```python
from build123d import *

# Parameters (mm, degrees)
F0_R        = 3.15
F1_DEPTH    = 6.5
F2_T1_DEPTH = 23.3593154951
F2_T3_DEPTH = 23.1607876028
F4_R        = 2


# Not quite as in the source:
# - a fillet or chamfer that OpenCascade refuses, or shapes differently, is made with other operations: its cross-section is extruded or revolved along the edge and cut away or added
# - two fillets or chamfers of one size are made in one step


with BuildPart() as f1:
    # F0 (on Top) → F1 (new body, symmetric)
    with BuildSketch(Plane.XY):
        with BuildLine():
            ThreePointArc((-2.7271020198, -1.7678842082), (-2.8555317961, 1.5519143538), (0, 3.25))
            Line((0, 3.25), (0, 9))
            Line((0, 9), (-35.4682957019, 7.5))
            Line((-35.4682957019, 7.5), (-34.834492885, -7.4866038177))
            Line((-34.834492885, -7.4866038177), (-24.8215810327, -7.0592907796))
            Line((-24.8215810327, -7.0592907796), (-25.0071863621, -2.7101377293))
            ThreePointArc((-25.0071863621, -2.7101377293), (-23.2018810758, 2.1742815392), (-19.0300843423, -0.9422535211))
            ThreePointArc((-19.0300843423, -0.9422535211), (-19.1270804103, -1.7303310583), (-19.4122789298, -2.4713683356))
            Line((-19.4122789298, -2.4713683356), (-19.2266736003, -6.8205213858))
            Line((-19.2266736003, -6.8205213858), (-2.5418620091, -6.1084770138))
            Line((-2.5418620091, -6.1084770138), (-2.7271020198, -1.7678842082))
        make_face()
        with BuildLine():
            ThreePointArc((3.25, 0), (3.153003932, -0.7880775372), (2.8678054126, -1.5291148144))
            Line((2.8678054126, -1.5291148144), (3.0586058071, -6))
            Line((3.0586058071, -6), (39.5, -6))
            Line((39.5, -6), (39.5, 9))
            Line((39.5, 9), (0, 9))
            Line((0, 9), (0, 3.25))
            ThreePointArc((0, 3.25), (2.2980970389, 2.2980970389), (3.25, 0))
        make_face()
        with Locations((31.9, 0)):
            Circle(F0_R, mode=Mode.SUBTRACT)
    extrude(amount=F1_DEPTH, both=True)

    # F2: chamfer of 2 x 1 on 4 edges, made by hand

    # F2_s2 → F2_t1 (cut)
    with BuildSketch(Plane.XY.offset(-11.6796577476)):
        Polygon((-24.9068558162, -5.0611095538), (-25.8206716456, -7.1019281713), (-24.8215810327, -7.0592907796), align=None)
        Polygon((-2.6271367926, -4.110295788), (-3.540952622, -6.1511144056), (-2.5418620091, -6.1084770138), align=None)
        Polygon((-18.2275829874, -6.7778839941), (-19.3119483838, -4.82234016), (-19.2266736003, -6.8205213858), align=None)
    extrude(amount=F2_T1_DEPTH, mode=Mode.SUBTRACT)

    # F2_s4 → F2_t3 (cut)
    with BuildSketch(Plane.XY.offset(-11.5803938014)):
        Polygon((3.97416362, -6), (2.9750730071, -4.0426373917), (3.0586058071, -6), align=None)
    extrude(amount=F2_T3_DEPTH, mode=Mode.SUBTRACT)

    # F4
    f4_edges = [f1.edges().sort_by_distance(p)[0] for p in [
        (-17.734148, 8.25, 6.5),
        (19.75, 9, 6.5),
        (-17.734148, 8.25, -6.5),
        (19.75, 9, -6.5),
        (-35.468296, 7.5, 0),
        (39.5, 9, 0),
        (39.5, 1.5, 6.5),
        (39.5, 1.5, -6.5),
        (-35.151394, 0.006698, -6.5),
        (-35.151394, 0.006698, 6.5),
        (-34.834493, -7.486604, 0),
        (-30.327582, -7.294266, -6.5),
        (-30.327582, -7.294266, 6.5),
        (-10.884268, -6.464499, 6.5),
        (-10.884268, -6.464499, -6.5),
        (21.737082, -6, 6.5),
        (39.5, -6, 0),
        (21.737082, -6, -6.5),
    ]]
    fillet(f4_edges, radius=F4_R)


solid = f1.part
```
The listing builds one solid part. Answer for the finished solid, in the listing's coordinates (mm). A direction names the side the tool comes from. Round coordinates to 2 decimals unless told otherwise and drop trailing zeros. Loops run counter-clockwise (first coordinate to the right, second up) from the corner with the lowest first, then second, coordinate; pieces in that order, holes last. Notation, with made-up numbers: (-15.5, 18) - (40.5, 18) arc R22 ccw to (40.5, 37) - close; hole circle Ø4 at (66.25, 73.5). An arc over 180 degrees is marked (long way). Use one line per item in the form item = value. Start each with the question number.
1. The part is cut by section D-D on z = -5.25. Determine the outline of the cut face in (x, y), then the cut area to 4 significant figures.
2. The part is cut by section C-C on y = 0. Give the number of separate pieces and of enclosed holes in the cut face, then the cut area to 3 significant figures.
3. The part is cut by section A-A on x = 31.9. Determine the outline of the cut face in (y, z), then the cut area to 3 significant figures.
4. A tool of negligible diameter and unlimited length cuts with its end or side. For faces 4 (the face through (-2.676, -2.955, 0.091)), 5 (the face through (2, 4, 6.5)), 6 (the face through (3.482, -5.035, -0.091)), from which of +Z, -Z, +X, -X, +Y, -Y can it reach the whole face along a straight path? Write none if from no direction.
5. Consider line 1 (X direction, y = 0.5, z = -2.25); line 2 (X direction, y = -4, z = 3.5); line 3 (X direction, y = 0.75, z = 1.75). Determine where each line is inside the solid, lowest interval first. Write a range as [from, to].
6. For a pull along X with two mould halves and no side action, classify faces 1 (the face through (21, -6, 0)), 2 (the face through (-19.363, -3.63, 0.091)), 3 (the face through (-29.377, -7.254, 0.063)) as pulls with the +X half, pulls with the -X half, needs draft (parallel to the pull), parting line crosses it, or undercut.
7. Given pin 1 Ø3 at (x, z) = (-9.5, -0.5) entering from +Y; pin 2 Ø1.5 at (x, y) = (3, -5) entering from -Z; pin 3 Ø2.5 at (x, z) = (21, -1) entering from -Y, each flat-ended and moving along its own axis, determine where each tip first touches the part or whether it passes through.
8. The part is cut by section B-B on z = 2. Determine the outline of the cut face in (x, y).
Geometry check:
q1.outline = (-35.24, 5.51) - (-34.77, -5.48) arc R1.85 ccw to (-32.84, -7.26) - (-25.75, -6.95) - (-24.91, -5.06) - (-25.01, -2.71) arc R3.25 cw (long way) to (-19.41, -2.47) - (-19.31, -4.82) - (-18.31, -6.64) - (-3.47, -6) - (-2.63, -4.11) - (-2.73, -1.77) arc R3.25 cw (long way) to (2.87, -1.53) - (2.98, -4.04) - (3.9, -5.85) - (37.5, -5.85) arc R1.85 ccw to (39.35, -4) - (39.35, 7) arc R1.85 ccw to (37.5, 8.85) - (0, 8.85) - (-33.46, 7.44) arc R1.85 ccw to start; hole circle Ø6.3 at (31.9, 0)
q1.area = 955.5 mm^2
q2.separate_pieces = 4
q2.enclosed_holes = 0
q2.area = 720 mm^2
q3.outline = (-6, -4.5) arc R2 ccw to (-4, -6.5) - (-3.15, -6.5) - (-3.15, 6.5) - (-4, 6.5) arc R2 ccw to (-6, 4.5) - close; (3.15, -6.5) - (7, -6.5) arc R2 ccw to (9, -4.5) - (9, 4.5) arc R2 ccw to (7, 6.5) - (3.15, 6.5) - close
q3.area = 110 mm^2
q4.face_4 = +Z, -Z
q4.face_5 = +Z, +X, -X, +Y, -Y
q4.face_6 = +Z, -Z, -Y
q5.line_1 = [-35.17, -25.19], [-19.37, -3.21], [3.21, 28.79], [35.01, 39.5]
q5.line_2 = [-34.98, -24.95], [-19.35, -2.63], [2.97, 39.5]
q5.line_3 = [-35.18, -25.05], [-19.51, -3.16], [3.16, 28.84], [34.96, 39.5]
q6.face_1 = needs draft
q6.face_2 = undercut
q6.face_3 = pulls with the +X half
q7.pin_1 = 8.66
q7.pin_2 = -6.48
q7.pin_3 = -6
q8.outline = (-35.38, 5.5) - (-34.92, -5.49) arc R2 ccw to (-32.84, -7.4) - (-25.82, -7.1) - (-24.91, -5.06) - (-25.01, -2.71) arc R3.25 cw (long way) to (-19.41, -2.47) - (-19.31, -4.82) - (-18.23, -6.78) - (-3.54, -6.15) - (-2.63, -4.11) - (-2.73, -1.77) arc R3.25 cw (long way) to (2.87, -1.53) - (2.98, -4.04) - (3.97, -6) - (37.5, -6) arc R2 ccw to (39.5, -4) - (39.5, 7) arc R2 ccw to (37.5, 9) - (0, 9) - (-33.47, 7.58) arc R2 ccw to start; hole circle Ø6.3 at (31.9, 0)
